For this review, take the finished solid that the model builds, in its own axes (mm). Face numbers are marked on the shaded views. A direction names the side the tool comes from. Coordinates: 2 decimals unless noted, no trailing zeros. Loops run counter-clockwise (first coordinate to the right, second up) from the corner with the lowest first, then second, coordinate; pieces in that order, holes last. Notation, with made-up numbers: (23.5, -23.5) -> (49.5, -23.5) arc R28 ccw to (49.5, 5.5) -> close; hole circle Ø3 at (-27, 65). An arc over 180 degrees is marked (long way). One line per item, written item: value.
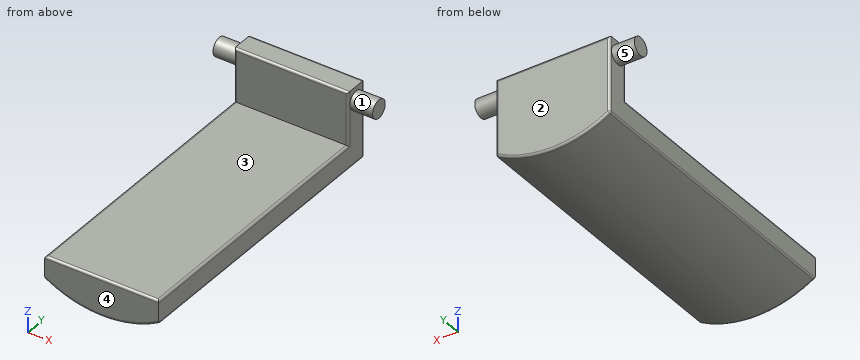
from build123d import *

# Parameters (mm, degrees)
SKETCH1_R                = 25
BOSS_EXTRUDE1_DEPTH      = 69
CUT_EXTRUDE3_DEPTH       = 69
SKETCH8_W                = 47.613521064
SKETCH8_H                = 96.094714493
CUT_EXTRUDE6_DEPTH       = 69
SKETCH9_W                = 16.650635095
SKETCH9_H                = 64
CUT_EXTRUDE7_DEPTH       = 69
SKETCH10_W               = 5
SKETCH10_H               = 9.23187044
CUT_EXTRUDE8_DEPTH       = 69
BOSS_EXTRUDE2_DEPTH      = 5
BOSS_EXTRUDE2_DEPTH_BACK = 30
SKETCH11_R               = 2
SKETCH12_W               = 21.924143589
SKETCH12_H               = 4
CUT_EXTRUDE9_DEPTH       = 80.284298572
FILLET1_R                = 0.5


with BuildPart() as part:
    # Sketch1 → Boss-Extrude1 (new body)
    with BuildSketch(Plane(origin=(0, 0, 0), x_dir=(1, 0, 0), z_dir=(0, 1, 0))):
        with Locations(Location((0, 0, 0), (0, 0, 270))):
            Circle(SKETCH1_R)
    extrude(amount=-BOSS_EXTRUDE1_DEPTH)

    # Sketch2 → Cut-Extrude3 (cut)
    with BuildSketch(Plane(origin=(0, 0, 0), x_dir=(1, 0, 0), z_dir=(0, 1, 0))):
        with BuildLine():
            Line((-12.5, -21.650635095), (-12.5, 21.650635095))
            ThreePointArc((-12.5, 21.650635095), (-25, 0), (-12.5, -21.650635095))
        make_face()
        with BuildLine():
            ThreePointArc((25, 0), (21.650635095, 12.5), (12.5, 21.650635095))
            Line((12.5, 21.650635095), (12.5, -21.650635095))
            ThreePointArc((12.5, -21.650635095), (21.650635095, -12.5), (25, 0))
        make_face()
    extrude(amount=-CUT_EXTRUDE3_DEPTH, mode=Mode.SUBTRACT)

    # Sketch8 → Cut-Extrude6 (cut)
    with BuildSketch(Plane(origin=(12.5, 0, 0), x_dir=(0, 0, -1), z_dir=(1, 0, 0))):
        with Locations((-23.806760532, -34.608459046)):
            Rectangle(SKETCH8_W, SKETCH8_H)
    extrude(amount=-CUT_EXTRUDE6_DEPTH, mode=Mode.SUBTRACT)

    # Sketch9 → Cut-Extrude7 (cut)
    with BuildSketch(Plane(origin=(12.5, 0, 0), x_dir=(0, 0, -1), z_dir=(1, 0, 0))):
        with Locations((8.325317548, -37)):
            Rectangle(SKETCH9_W, SKETCH9_H)
    extrude(amount=-CUT_EXTRUDE7_DEPTH, mode=Mode.SUBTRACT)

    # Sketch10 → Cut-Extrude8 (cut)
    with BuildSketch(Plane(origin=(12.5, 0, 0), x_dir=(0, 0, -1), z_dir=(1, 0, 0))):
        with Locations((2.5, -4.61593522)):
            Rectangle(SKETCH10_W, SKETCH10_H)
    extrude(amount=-CUT_EXTRUDE8_DEPTH, mode=Mode.SUBTRACT)

    # Sketch11 → Boss-Extrude2 (add, two sides: drawn at the far end of the back side and taken through both)
    with BuildSketch(Plane(origin=(12.5, 0, 0), x_dir=(0, 0, -1), z_dir=(1, 0, 0)).offset(-BOSS_EXTRUDE2_DEPTH_BACK)):
        with Locations((8, -2.5)):
            Circle(SKETCH11_R)
    extrude(amount=BOSS_EXTRUDE2_DEPTH + BOSS_EXTRUDE2_DEPTH_BACK)

    # Sketch12 → Cut-Extrude9 (cut, through all)
    with BuildSketch(Plane(origin=(12.5, 0, 0), x_dir=(0, 0, -1), z_dir=(1, 0, 0))):
        with Locations((27.61270689, -67)):
            Rectangle(SKETCH12_W, SKETCH12_H)
    extrude(amount=-CUT_EXTRUDE9_DEPTH, mode=Mode.SUBTRACT)

    # Fillet1
    fillet1_edges = [part.edges().sort_by_distance(p)[0] for p in [
        (12.5, -35, -16.650635095),
        (0, -65, -16.650635095),
        (-12.5, -32.5, -21.650635095),
        (12.5, -32.5, -21.650635095),
        (0, -65, -25),
        (-12.5, 0, -13.325317547),
        (12.5, 0, -13.325317547),
        (-12.5, -35, -16.650635095),
        (12.5, -5, -10.825317547),
        (0, 0, -25),
        (-12.5, -5, -10.825317547),
        (0, -5, -5),
        (0, 0, -5),
    ]]
    fillet(fillet1_edges, radius=FILLET1_R - 0.0001)  # a hair under: the kernel refuses the full size


solid = part.part
1. Insertion check: pin 1 Ø8 at (y, z) = (-23.5, -15.5) entering from +X; pin 2 Ø5 at (y, z) = (-20.5, -14.5) entering from -X; pin 3 Ø1.5 at (y, z) = (-54.5, -14) entering from -X; pin 4 Ø7 at (x, y) = (4, -31) entering from +Z. Each pin has a flat end and moves straight along its axis. Give the tip position at first contact, or say it passes through.
Return value:
pin 1: stops at x = 12.5
pin 2: stops at x = -12.48
pin 3: passes through
pin 4: stops at z = -16.65
2. To check wall thickness, follow probe 1 along X at (y, z) = (-55.5, -17.5); probe 2 along Y at (x, z) = (-6.5, -11); probe 3 along Z at (x, y) = (-5, -25). State the ranges of each line that lie inside material, in increasing order. Write a range as from..to.
Return value:
probe 1: x = -12.5..12.5
probe 2: y = -5..0
probe 3: z = -24.49..-16.65
3. Take a section at C-C, the plane x = 15. Give the boundary of the cut face in (y, z), and give its area (3 significant figures).
Return value:
outline: circle Ø4 at (-2.5, -8)
area: 12.6 mm2
4. Take a section at A-A, the plane y = -21.5. Give the boundary of the cut face in (x, z), and give its area (3 significant figures).
Return value:
outline: (-12.5, -21.36) arc R0.5 ccw to (-12.24, -21.8) arc R25 ccw to (12.24, -21.8) arc R0.5 ccw to (12.5, -21.36) -> (12.5, -17.15) arc R0.5 ccw to (12, -16.65) -> (-12, -16.65) arc R0.5 ccw to (-12.5, -17.15) -> close
area: 181 mm2
5. Take a section at D-D, the plane y = -2.5. Give the boundary of the cut face in (x, z).
Return value:
outline: (-17.5, -10) -> (-12.5, -10) -> (-12.5, -21.36) arc R0.5 ccw to (-12.24, -21.8) arc R25 ccw to (12.24, -21.8) arc R0.5 ccw to (12.5, -21.36) -> (12.5, -10) -> (17.5, -10) -> (17.5, -6) -> (12.5, -6) -> (12.5, -5) -> (-12.5, -5) -> (-12.5, -6) -> (-17.5, -6) -> close
6. For the marked faces 1, 2, 3, 4 and 5, list the 3-axis set-ups (+Z, -Z, +X, -X, +Y, -Y) from which the entire face can be reached by the end or side of a thin tool; tool diameter is ignored.
Return value:
face 1: +X
face 2: +Z, -Z, +X, -X, +Y
face 3: +Z, +X, -X, -Y
face 4: +Z, -Z, +X, -X, -Y
face 5: -X
